```python
from build123d import *

# Parameters (mm, degrees)
SKETCH1_R               = 76.2
BOSS_EXTRUDE1_DEPTH     = 3.81
SKETCH2_R               = 0.7366
CUT_EXTRUDE1_DEPTH      = 108.830404339
CIRPATTERN1_COUNT       = 6
SKETCH3_R               = 6.35
CUT_EXTRUDE2_DEPTH      = 108.830404339
SKETCH5_R               = 3.175
CUT_EXTRUDE3_DEPTH      = 108.830404339
CIRPATTERN2_COUNT       = 8
SKETCH6_W               = 1.27
SKETCH6_H               = 2.54
CUT_EXTRUDE4_DEPTH      = 108.830404339
CUT_EXTRUDE4_DEPTH_BACK = 108.830404339
SKETCH7_R               = 76.2
SKETCH7_R_2             = 31.75


with BuildPart() as part:
    # Sketch1 → Boss-Extrude1 (new body)
    with BuildSketch(Plane.XY):
        with Locations(Location((0, 0, 0), (0, 0, 180))):
            Circle(SKETCH1_R)
    extrude(amount=BOSS_EXTRUDE1_DEPTH)

    # Sketch2 → Cut-Extrude1 (cut, through all)
    with BuildSketch(Plane(origin=(0, 0, 0), x_dir=(-1, 0, 0), z_dir=(0, 0, -1))):
        with Locations((0, 10.16)):
            Circle(SKETCH2_R)
        with Locations((2.54, 14.559409051)):
            Circle(SKETCH2_R)
        with Locations((5.08, 10.16)):
            Circle(SKETCH2_R)
        with Locations((7.62, 14.559409051)):
            Circle(SKETCH2_R)
        with Locations((-2.54, 14.559409051)):
            Circle(SKETCH2_R)
        with Locations((-5.08, 18.958818102)):
            Circle(SKETCH2_R)
        with Locations((0, 18.958818102)):
            Circle(SKETCH2_R)
        with Locations((5.08, 18.958818102)):
            Circle(SKETCH2_R)
    cut_extrude1 = extrude(amount=-CUT_EXTRUDE1_DEPTH, mode=Mode.SUBTRACT)

    # CirPattern1: Cut-Extrude1 ×6 about axis
    cirpattern1_axis = Axis((0, 0, 0), (0, 0, 1))
    for i in range(1, CIRPATTERN1_COUNT):
        add(cut_extrude1.rotate(cirpattern1_axis, i * 360 / CIRPATTERN1_COUNT), mode=Mode.SUBTRACT)

    # Sketch3 → Cut-Extrude2 (cut, through all)
    with BuildSketch(Plane(origin=(0, 0, 0), x_dir=(-1, 0, 0), z_dir=(0, 0, -1))):
        with Locations((41.275, 0)):
            Circle(SKETCH3_R)
        with Locations((-41.275, 0)):
            Circle(SKETCH3_R)
    extrude(amount=-CUT_EXTRUDE2_DEPTH, mode=Mode.SUBTRACT)

    # Sketch5 → Cut-Extrude3 (cut, through all)
    with BuildSketch(Plane(origin=(0, 0, 0), x_dir=(-1, 0, 0), z_dir=(0, 0, -1))):
        with Locations((66.802, 0)):
            Circle(SKETCH5_R)
    cut_extrude3 = extrude(amount=-CUT_EXTRUDE3_DEPTH, mode=Mode.SUBTRACT)

    # CirPattern2: Cut-Extrude3 ×8 about axis
    cirpattern2_axis = Axis((0, 0, 0), (0, 0, 1))
    for i in range(1, CIRPATTERN2_COUNT):
        add(cut_extrude3.rotate(cirpattern2_axis, i * 360 / CIRPATTERN2_COUNT), mode=Mode.SUBTRACT)

    # Sketch6 → Revolve1 (revolve)
    with BuildSketch(Plane(origin=(0, 0, 0), x_dir=(0, 0, -1), z_dir=(1, 0, 0))):
        with Locations((0.635, 52.07)):
            Rectangle(SKETCH6_W, SKETCH6_H)
    revolve(axis=Axis((0, 0, 0), (0, 0, 1)))

    # Sketch7 → Cut-Extrude4 (cut, two sides: drawn at the far end of the back side and taken through both)
    with BuildSketch(Plane.XY.offset(-CUT_EXTRUDE4_DEPTH_BACK)):
        Circle(SKETCH7_R)
        with Locations(Location((0, 0, 0), (0, 0, 180))):
            Circle(SKETCH7_R_2, mode=Mode.SUBTRACT)
    extrude(amount=CUT_EXTRUDE4_DEPTH + CUT_EXTRUDE4_DEPTH_BACK, mode=Mode.SUBTRACT)


solid = part.part
```
The listing builds one solid part. Answer for the finished solid, in the listing's coordinates (mm). Coordinates: 2 decimals unless noted, no trailing zeros. Write each loop counter-clockwise with the first axis right and the second up, starting at its lowest first coordinate (ties: lowest second). Pieces come first, ordered by that corner, then holes. Notation, with made-up numbers: M 37,27 L 68,27 A17 ccw 68,46 Z; hole C 6.25,-12 d8. An arc over 180 degrees is marked long. Use a Markdown table: item, result. Add a question column.
1. Given P1, Ø0.9, axis at x = -5.08, y = 18.96, coming from the -Z side; P2, Ø1.5, axis at x = 18, z = 3, coming from the -Y side, each flat-ended and moving along its own axis, determine where each tip first touches the part or whether it passes through.
2. Section C-C (z = 1.7) is taken. Count the separate pieces of the cut face and the enclosed holes in it, plus the area to 3 significant figures.
3. Section D-D (x = 25) is taken. Give the vertices of the cut face in (y, z).
4. Straight lines are drawn through the part: line 1 along Y through (x, z) = (-5.08, 3.05); line 2 along Y through (x, z) = (5.08, 2.25); line 3 along X through (y, z) = (10.5, 1.45). For each, find the intervals that lie inside material, in ascending order. Write a range as [from, to].
5. For a pull along Y with two mould halves and no side action, classify faces 1 (the flat face through (0, 0, 3.81)), 2 (the cylindrical face through (-0.1, -19.69, 1.88)) as +Y half, -Y half, draft (parallel to the pull), parting line (faces both ways), or undercut.
6. Section B-B (y = -8) is taken. Give the vertices of the cut face in (x, z), plus the area to 3 significant figures.
7. Section A-A (x = 2.54) is taken. Give the vertices of the cut face in (y, z), plus the area to 3 significant figures.
Data:
| question | item | result |
|---|---|---|
| 1 | P1 | passes through |
| 1 | P2 | stops at y = -26.66 |
| 2 | separate pieces | 1 |
| 2 | enclosed holes | 48 |
| 2 | area | 3,090 mm2 |
| 3 | outline | M -19.57,0 L 19.57,0 L 19.57,3.81 L -19.57,3.81 Z |
| 4 | line 1 | y = [-31.34, -19.7], [-18.22, 9.42], [10.9, 18.22], [19.7, 31.34] |
| 4 | line 2 | y = [-31.34, -19.7], [-18.22, -10.9], [-9.42, 18.22], [19.7, 31.34] |
| 4 | line 3 | x = [-29.96, -5.73], [-4.43, -0.65], [0.65, 29.96] |
| 5 | face 1 | draft |
| 5 | face 2 | undercut |
| 6 | outline | M -30.73,0 L 30.73,0 L 30.73,3.81 L -30.73,3.81 Z |
| 6 | area | 234 mm2 |
| 7 | outline | M -31.65,0 L -15.3,0 L -15.3,3.81 L -31.65,3.81 Z; M -13.82,0 L 13.82,0 L 13.82,3.81 L -13.82,3.81 Z; M 15.3,0 L 31.65,0 L 31.65,3.81 L 15.3,3.81 Z |
| 7 | area | 230 mm2 |
